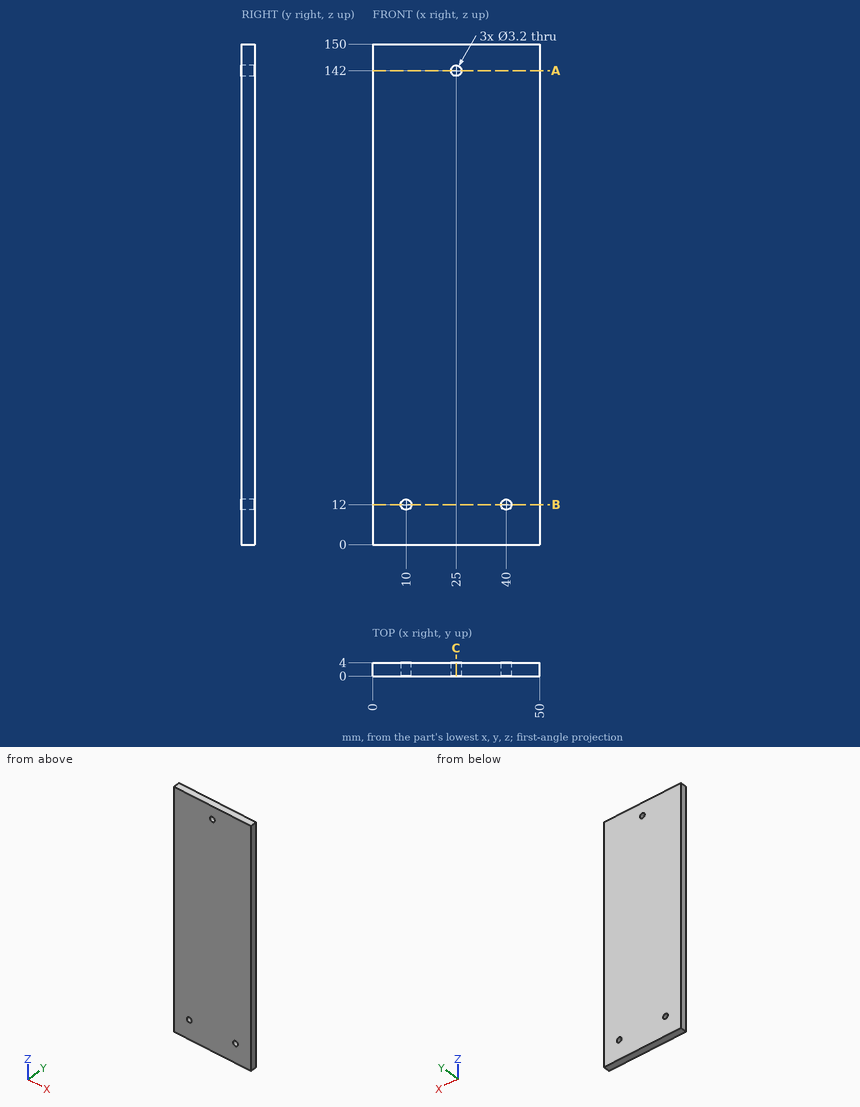
The figure shows three views and two pictorial views of one solid part (mm, origin at its lowest corner). Answer the questions. Give positions to 0.01 mm unless a question says otherwise; leave off trailing zeros. Write each loop counter-clockwise with the first axis right and the second up, starting at its lowest first coordinate (ties: lowest second). Pieces come first, ordered by that corner, then holes. Notation, with made-up numbers: (56.5, -15) - (63.5, -15) arc R12 ccw to (63.5, 6) - close; hole circle Ø10 at (13, 67.5). An arc over 180 degrees is marked (long way). Use one line per item in the form item = value.
1. A cutting plane is placed at B-B (z = 12). Write down the section's boundary in (x, y).
Filled in:
outline = (0, 0) - (8.4, 0) - (8.4, 4) - (0, 4) - close; (11.6, 0) - (38.4, 0) - (38.4, 4) - (11.6, 4) - close; (41.6, 0) - (50, 0) - (50, 4) - (41.6, 4) - close
2. A cutting plane is placed at C-C (x = 25). Write down the section's boundary in (y, z), and give its area (3 significant figures).
Filled in:
outline = (0, 0) - (4, 0) - (4, 140.4) - (0, 140.4) - close; (0, 143.6) - (4, 143.6) - (4, 150) - (0, 150) - close
area = 587 mm^2
3. Consider L1, parallel to X at y = 3.15, z = 12; L2, parallel to X at y = 1.85, z = 142; L3, parallel to Z at x = 10, y = 2.8. Determine where each line is inside the solid, lowest interval first.
Filled in:
L1 = 0 to 8.4, 11.6 to 38.4, 41.6 to 50
L2 = 0 to 23.4, 26.6 to 50
L3 = 0 to 10.4, 13.6 to 150
4. This flat-tipped pin is pushed along its axis until it touches: pin 1 Ø1 at (y, z) = (3.5, 39.5) entering from -X. Where does it stop, or does it pass through?
Filled in:
pin_1 = 0
5. A cutting plane is placed at A-A (z = 142). Write down the section's boundary in (x, y), and give its area (3 significant figures).
Filled in:
outline = (0, 0) - (23.4, 0) - (23.4, 4) - (0, 4) - close; (26.6, 0) - (50, 0) - (50, 4) - (26.6, 4) - close
area = 187 mm^2
